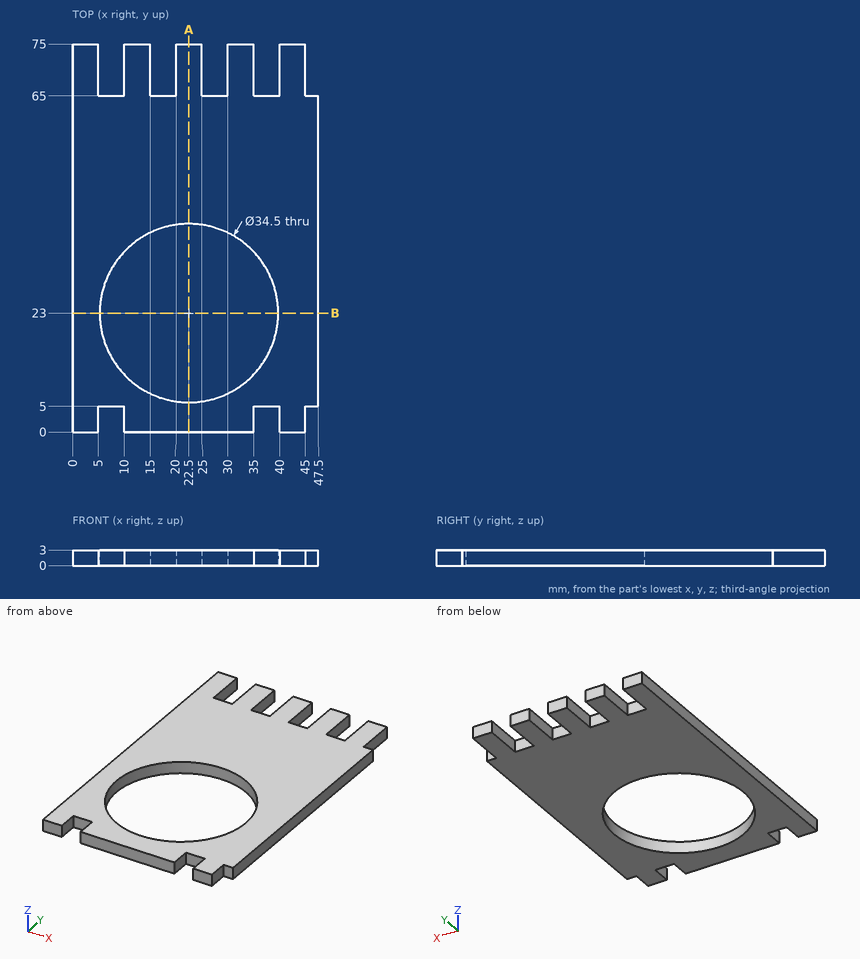
Input: dimensioned drawing with shaded views. Units: mm. Origin: part minimum x, y, z. Give positions to 0.01 mm unless a question says otherwise; leave off trailing zeros. Write each loop counter-clockwise with the first axis right and the second up, starting at its lowest first coordinate (ties: lowest second). Pieces come first, ordered by that corner, then holes. Notation, with made-up numbers: (-27, 88.5) - (-20, 88.5) arc R22 cw to (-20, 97.5) - close; hole circle Ø10 at (6, 50.5). An arc over 180 degrees is marked (long way). One line per item, written item: value. Start each with the question number.
Q1. Material intervals for probe 1 along X at (y, z) = (66.5, 1.65); probe 2 along X at (y, z) = (4.5, 1.95); probe 3 along Y at (x, z) = (22.5, 0.85), sorted ascending. Write a range as from..to.
Q2. Section query A-A, the plane x = 22.5. Return the cut outline in (y, z).
Q3. First-contact query: pin 1 Ø1 at (x, z) = (27.5, 2.5) entering from +Y. Flat tip, straight axial feed; report the tip coordinate or a pass-through.
Q4. Section query B-B, the plane y = 23. Return the cut outline in (x, z), then the cut area to 3 significant figures.
Answer:
1. probe 1: x = 0..5, 10..15, 20..25, 30..35, 40..45
1. probe 2: x = 0..5, 10..35, 40..45
1. probe 3: y = 0..5.75, 40.25..75
2. outline: (0, 0) - (5.75, 0) - (5.75, 3) - (0, 3) - close; (40.25, 0) - (75, 0) - (75, 3) - (40.25, 3) - close
3. pin 1: stops at y = 65
4. outline: (0, 0) - (5.25, 0) - (5.25, 3) - (0, 3) - close; (39.75, 0) - (47.5, 0) - (47.5, 3) - (39.75, 3) - close
4. area: 39.0 mm2
